Can you work these out from the drawing? Everything is in mm from the part's minimum corner. A direction names the side the tool comes from. Coordinates: 2 decimals unless noted, no trailing zeros. Loops run counter-clockwise (first coordinate to the right, second up) from the corner with the lowest first, then second, coordinate; pieces in that order, holes last.
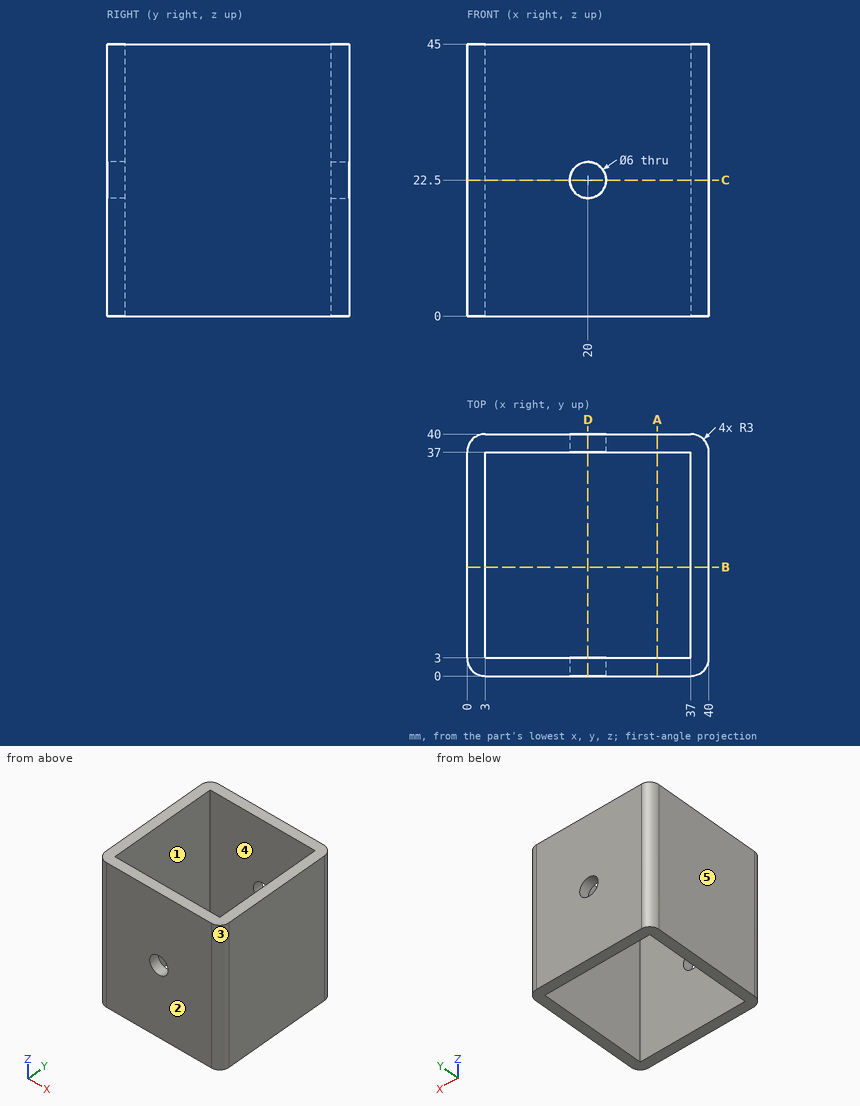
(1) We'd pull the mould along X, two halves only. Please class the marked faces 3, 4 and 5: +X half, -X half, draft (parallel to the pull), parting line (faces both ways), or undercut.
Answers:
face 3: +X half
face 4: undercut
face 5: -X half
(2) Which directions (+Z, -Z, +X, -X, +Y, -Y) give clear straight access to the entire face, cutting with the end or side of a thin tool? Please do the marked faces 1 and 2.
Answers:
face 1: +Z, -Z
face 2: +Z, -Z, +X, -X, -Y
(3) Imagine slicing it at D-D, the plane x = 20. Write out the boundary of the cut face in (y, z), and give its area (3 significant figures).
Answers:
outline: (0, 0) - (3, 0) - (3, 19.5) - (0, 19.5) - close; (0, 25.5) - (3, 25.5) - (3, 45) - (0, 45) - close; (37, 0) - (40, 0) - (40, 19.5) - (37, 19.5) - close; (37, 25.5) - (40, 25.5) - (40, 45) - (37, 45) - close
area: 234 mm2
(4) Imagine slicing it at C-C, the plane z = 22.5. Write out the boundary of the cut face in (x, y), and give its area (3 significant figures).
Answers:
outline: (0, 3) arc R3 ccw to (3, 0) - (17, 0) - (17, 3) - (3, 3) - (3, 37) - (17, 37) - (17, 40) - (3, 40) arc R3 ccw to (0, 37) - close; (23, 0) - (37, 0) arc R3 ccw to (40, 3) - (40, 37) arc R3 ccw to (37, 40) - (23, 40) - (23, 37) - (37, 37) - (37, 3) - (23, 3) - close
area: 400 mm2
(5) For pin 1 (9.5 mm diameter, centred on x = 20, z = 22.5, fed in from -Y); pin 2 (5 mm diameter, centred on x = 20, z = 22.5, fed in from +Y), each with a flat end and sliding along its axis, tell me the tip position at first contact or that it passes through.
Answers:
pin 1: stops at y = 0
pin 2: passes through
(6) I need wall thicknesses on probe 1 along Y at (x, z) = (11, 28.5); probe 2 along Z at (x, y) = (20, 2.2). Which ranges of each line are inside material? Lowest first, please.
Answers:
probe 1: y = 0 to 3, 37 to 40
probe 2: z = 0 to 19.5, 25.5 to 45
(7) Imagine slicing it at A-A, the plane x = 31.5. Write out the boundary of the cut face in (y, z).
Answers:
outline: (0, 0) - (3, 0) - (3, 45) - (0, 45) - close; (37, 0) - (40, 0) - (40, 45) - (37, 45) - close
